```python
from build123d import *

# Parameters (mm, degrees)
F0_R      = 32.5
F1_DEPTH  = 10
F2_R      = 15.5
F3_DEPTH  = 35
F5_R      = 4.8
F6_DEPTH  = 45.001
F7_R      = 4.8
F8_DEPTH  = 34
F10_DEPTH = 22
F12_DEPTH = 6
F13_R     = 2.1
F14_DEPTH = 25
F15_R     = 3.25
F16_DEPTH = 45.0010001
F17_R     = 3.25
F18_DEPTH = 2.5


# Not quite as in the source:
# - a feature names something its author has since deleted; it is built from what else it names


with BuildPart() as f1:
    # F0 (on Top) → F1 (new body)
    with BuildSketch(Plane.XY):
        Circle(F0_R)
    extrude(amount=F1_DEPTH)

    # F2 (on face) → F3 (join)
    with BuildSketch(Plane.XY.offset(10)):
        Circle(F2_R)
    extrude(amount=F3_DEPTH)

    # F5 (on face) → F6 (cut, through all)
    with BuildSketch(Plane.XY):
        Circle(F5_R)
    extrude(amount=F6_DEPTH, mode=Mode.SUBTRACT)

    # F7 (on face) → F8 (cut)
    with BuildSketch(Plane.XY.offset(45)):
        Polygon((3.3412309145, -6.2007668324), (7.040637057, -0.2067925644), (3.6994061426, 5.993974268), (-3.3412309145, 6.2007668324), (-7.040637057, 0.2067925644), (-3.6994061426, -5.993974268), align=None)
        Circle(F7_R, mode=Mode.SUBTRACT)
    extrude(amount=-F8_DEPTH, mode=Mode.SUBTRACT)

    # F9 (on face) → F10 (cut)
    with BuildSketch(Plane.XY.offset(45)):
        Polygon((-4.4167295593, -7.65), (4.4167295593, -7.65), (8.8334591186, 0), (4.4167295593, 7.65), (-4.4167295593, 7.65), (-8.8334591186, 0), align=None)
        Polygon((3.3412309145, -6.2007668324), (-3.6994061426, -5.993974268), (-7.040637057, 0.2067925644), (-3.3412309145, 6.2007668324), (3.6994061426, 5.993974268), (7.040637057, -0.2067925644), align=None, mode=Mode.SUBTRACT)
    extrude(amount=-F10_DEPTH, mode=Mode.SUBTRACT)

    # F11 (on face) → F12 (cut)
    with BuildSketch(Plane.XY):
        Polygon((-15.35, -8.8623266321), (-20.5, -5.8889727457), (-25.65, -8.8623266321), (-25.65, -14.8090344047), (-20.5, -17.782388291), (-15.35, -14.8090344047), align=None)
        Polygon((0, 29.6180688094), (-5.15, 26.6447149231), (-5.15, 20.6980071504), (0, 17.7246532641), (5.15, 20.6980071504), (5.15, 26.6447149231), align=None)
        Polygon((25.65, -14.8090344047), (25.65, -8.8623266321), (20.5, -5.8889727457), (15.35, -8.8623266321), (15.35, -14.8090344047), (20.5, -17.782388291), align=None)
    extrude(amount=F12_DEPTH, mode=Mode.SUBTRACT)

    # F13 (on Right) → F14 (cut, symmetric)
    with BuildSketch(Plane.YZ):
        with Locations((0, 29)):
            Circle(F13_R)
    extrude(amount=F14_DEPTH, both=True, mode=Mode.SUBTRACT)

    # F15 (on face) → F16 (cut, through all)
    with BuildSketch(Plane.XY):
        with Locations((-20.5, -11.8356805184)):
            Circle(F15_R)
        with Locations((0, 23.6713610368)):
            Circle(F15_R)
        with Locations((20.5, -11.8356805184)):
            Circle(F15_R)
    extrude(amount=F16_DEPTH, mode=Mode.SUBTRACT)

    # F17 (on face) → F18 (cut)
    with BuildSketch(Plane.XY):
        with BuildLine():
            ThreePointArc((-25.1062968267, -16.4217495916), (-18.0191664076, -17.8436306419), (-14, -11.8356805184))
            ThreePointArc((-14, -11.8356805184), (-21.3555101482, -5.3922262905), (-26.7748007343, -13.5318160511))
            ThreePointArc((-26.7748007343, -13.5318160511), (-25.9807621135, -15), (-25.1062968267, -16.4217495916))
        make_face()
        with Locations((-20.5, -11.8356805184)):
            Circle(F17_R, mode=Mode.SUBTRACT)
        with BuildLine():
            ThreePointArc((-25.1062968267, -16.4217495916), (-25.9807621135, -15), (-26.7748007343, -13.5318160511))
            ThreePointArc((-26.7748007343, -13.5318160511), (-26.1291651246, -15.0856805184), (-25.1062968267, -16.4217495916))
        make_face()
        with BuildLine():
            ThreePointArc((1.6685039075, 29.9535656427), (0, 30), (-1.6685039075, 29.9535656427))
            ThreePointArc((-1.6685039075, 29.9535656427), (-3.9626206354, 18.5189210614), (6.5, 23.6713610368))
            ThreePointArc((6.5, 23.6713610368), (5.1524399753, 27.6339816722), (1.6685039075, 29.9535656427))
        make_face()
        with BuildLine():
            ThreePointArc((1.6685039075, 29.9535656427), (0, 30.1713610368), (-1.6685039075, 29.9535656427))
            ThreePointArc((-1.6685039075, 29.9535656427), (0, 30), (1.6685039075, 29.9535656427))
        make_face()
        with BuildLine():
            ThreePointArc((26.7748007343, -13.5318160511), (25.9807621135, -15), (25.1062968267, -16.4217495916))
            ThreePointArc((25.1062968267, -16.4217495916), (26.1291651246, -15.0856805184), (26.7748007343, -13.5318160511))
        make_face()
        with BuildLine():
            ThreePointArc((27, -11.8356805184), (14.4920498765, -9.354846926), (25.1062968267, -16.4217495916))
            ThreePointArc((25.1062968267, -16.4217495916), (25.9807621135, -15), (26.7748007343, -13.5318160511))
            ThreePointArc((26.7748007343, -13.5318160511), (26.9434542278, -12.6911906666), (27, -11.8356805184))
        make_face()
    extrude(amount=F18_DEPTH, mode=Mode.SUBTRACT)


solid = f1.part
```
Could you check a few things on this model? Use its own coordinates, in mm. A direction names the side the tool comes from. Round coordinates to 2 decimals unless told otherwise and drop trailing zeros. Order: outer loops, then holes, each group sorted by start corner. A loop starts at its lowest first (then second) coordinate and runs counter-clockwise, first axis right, second up. Notation, with made-up numbers: (-3, 30) -> (30, 30) arc R29 cw to (30, 63) -> close; hole circle Ø8 at (-37.5, -5.5). An arc over 180 degrees is marked (long way). One line per question, with ' | ' between items.
Q1. If we section it at C-C on z = 9: Write out the boundary of the cut face in (x, y), plus the area to 3 significant figures.
Computed values:
outline: circle Ø65 at (0, 0); hole circle Ø6.5 at (-20.5, -11.84); hole circle Ø9.6 at (0, 0); hole circle Ø6.5 at (0, 23.67); hole circle Ø6.5 at (20.5, -11.84) | area: 3,150 mm²
Q2. If we section it at B-B on x = -10: Write out the boundary of the cut face in (y, z), plus the area to 3 significant figures.
Computed values:
outline: (-30.92, 0) -> (30.92, 0) -> (30.92, 10) -> (11.84, 10) -> (11.84, 45) -> (-11.84, 45) -> (-11.84, 10) -> (-30.92, 10) -> close; hole circle Ø4.2 at (0, 29) | area: 1,430 mm²
Q3. If we section it at D-D on z = 29: Write out the boundary of the cut face in (x, y), plus the area to 3 significant figures.
Computed values:
outline: (-15.36, -2.1) arc R15.5 ccw to (15.36, -2.1) -> (7.62, -2.1) -> (4.42, -7.65) -> (-4.42, -7.65) -> (-7.62, -2.1) -> close; (-15.36, 2.1) -> (-7.62, 2.1) -> (-4.42, 7.65) -> (4.42, 7.65) -> (7.62, 2.1) -> (15.36, 2.1) arc R15.5 ccw to start | area: 491 mm²
Q4. I'm going to push flat-ended pins straight in: pin 1 (1 mm diameter, centred on x = -0.5, y = -5, fed in from +Z); pin 2 (4 mm diameter, centred on y = -13, z = 4, fed in from +X); pin 3 (5 mm diameter, centred on y = 7, z = 16, fed in from -X); pin 4 (7.5 mm diameter, centred on x = 0, y = 0, fed in from +Z). Where does each tip first touch, or does it pass through?
Computed values:
pin 1: z = 11 | pin 2: x = 30.58 | pin 3: x = -14.83 | pin 4: through
Q5. We'd pull the mould along Y, two halves only. Please class faces 1 (the face through (-15.35, -12, 4)), 2 (the face through (31, 9.76, 4.93)), 3 (the face through (-7, 4, 45)): released by +Y, released by -Y, zero draft, split by the parting line, or undercut.
Computed values:
face 1: undercut | face 2: split by the parting line | face 3: zero draft
Q6. Which directions (+Z, -Z, +X, -X, +Y, -Y) give clear straight access to the entire face, cutting with the end or side of a thin tool? Please do faces 4 (the face through (11.62, -2.1, 29.09)), 5 (the face through (-6.656, -3.771, 34.154)), 6 (the face through (-23.111, -16.275, 4.226)).
Computed values:
face 4: +X, -X | face 5: +Z | face 6: -Z
Q7. If I drill on line 1 (Y direction, x = 0, z = 2.75); line 2 (Z direction, x = 13, y = 0); line 3 (Y direction, x = -20.5, z = 1.9), over which ranges is the centre line in solid material (lowest first)? Write a range as from..to.
Computed values:
line 1: -32.5..-4.8, 4.8..17.72, 29.62..32.5 | line 2: 0..26.9, 31.1..45 | line 3: -25.22..-18.34, -5.34..25.22
Q8. If we section it at A-A on z = 19.5: Write out the boundary of the cut face in (x, y).
Computed values:
outline: circle Ø31 at (0, 0); hole (-7.04, 0.21) -> (-3.7, -5.99) -> (3.34, -6.2) -> (7.04, -0.21) -> (3.7, 5.99) -> (-3.34, 6.2) -> close
